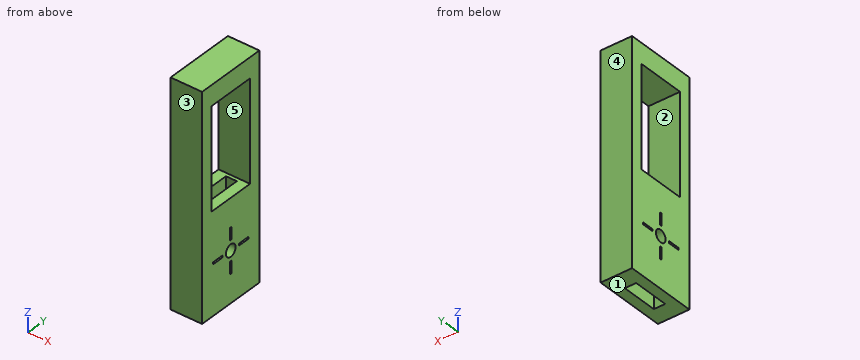
```python
from build123d import *

# Parameters (mm, degrees)
SKETCH1_W           = 17.8
SKETCH1_H           = 25
SKETCH1_R           = 1.5
BOSS_EXTRUDE1_DEPTH = 3.9
SKETCH3_W           = 0.5
SKETCH3_H           = 3
CUT_EXTRUDE1_DEPTH  = 10
CIRPATTERN1_COUNT   = 4
SKETCH4_W           = 2.7
SKETCH4_H           = 10.2
CUT_EXTRUDE2_DEPTH  = 18
SKETCH5_W           = 2.8
SKETCH5_H           = 9
CUT_EXTRUDE3_DEPTH  = 10
SKETCH6_W           = 7.8
SKETCH6_H           = 17.8
BOSS_EXTRUDE2_DEPTH = 30
SKETCH7_W           = 25
SKETCH7_H           = 12
CUT_EXTRUDE4_DEPTH  = 30


with BuildPart() as part:
    # Sketch1 → Boss-Extrude1 (new, symmetric)
    with BuildSketch(Plane.YZ):
        Rectangle(SKETCH1_W, SKETCH1_H)
        with Locations(Location((0, 0, 0), (0, 0, 270))):
            Circle(SKETCH1_R, mode=Mode.SUBTRACT)
    extrude(amount=BOSS_EXTRUDE1_DEPTH, both=True)

    # Sketch3 → Cut-Extrude1 (cut)
    with BuildSketch(Plane(origin=(3.9, 0, 0), x_dir=(0, 0, -1), z_dir=(1, 0, 0))):
        with Locations((0, 4)):
            Rectangle(SKETCH3_W, SKETCH3_H)
    cut_extrude1 = extrude(amount=-CUT_EXTRUDE1_DEPTH, mode=Mode.SUBTRACT)

    # CirPattern1: Cut-Extrude1 ×4 about axis
    cirpattern1_axis = Axis((0, 0, 0), (1, 0, 0))
    for i in range(1, CIRPATTERN1_COUNT):
        add(cut_extrude1.rotate(cirpattern1_axis, i * 360 / CIRPATTERN1_COUNT), mode=Mode.SUBTRACT)

    # Sketch4 → Cut-Extrude2 (cut)
    with BuildSketch(Plane.XY.offset(12.5)):
        Rectangle(SKETCH4_W, SKETCH4_H)
    extrude(amount=-CUT_EXTRUDE2_DEPTH, mode=Mode.SUBTRACT)

    # Sketch5 → Cut-Extrude3 (cut)
    with BuildSketch(Plane(origin=(0, 0, -12.5), x_dir=(-1, 0, 0), z_dir=(0, 0, -1))):
        Rectangle(SKETCH5_W, SKETCH5_H)
    extrude(amount=-CUT_EXTRUDE3_DEPTH, mode=Mode.SUBTRACT)

    # Sketch6 → Boss-Extrude2 (add)
    with BuildSketch(Plane.XY.offset(12.5)):
        Rectangle(SKETCH6_W, SKETCH6_H)
    extrude(amount=BOSS_EXTRUDE2_DEPTH)

    # Sketch7 → Cut-Extrude4 (cut)
    with BuildSketch(Plane(origin=(3.9, 0, 0), x_dir=(0, 0, -1), z_dir=(1, 0, 0))):
        with Locations((-25, 0)):
            Rectangle(SKETCH7_W, SKETCH7_H)
    extrude(amount=-CUT_EXTRUDE4_DEPTH, mode=Mode.SUBTRACT)


solid = part.part
```
Can you work these out from the model? Positions are in its coordinate system, mm. Face numbers are marked on the shaded views. A direction names the side the tool comes from. Coordinates: 2 decimals unless noted, no trailing zeros. Loops run counter-clockwise (first coordinate to the right, second up) from the corner with the lowest first, then second, coordinate; pieces in that order, holes last. Notation, with made-up numbers: M -7,37 L 0,37 A14 cw 0,43 Z; hole C 75,25 d1. An arc over 180 degrees is marked long. Put each result on its own line as item: value. Start each with the question number.
(1) I need wall thicknesses on probe 1 along Z at (x, y) = (-1.5, 3.75); probe 2 along Y at (x, z) = (3.15, 0); probe 3 along Y at (x, z) = (-2.25, 28.5). Which ranges of each line are inside material? Lowest first, please.
(2) Which directions (+Z, -Z, +X, -X, +Y, -Y) give clear straight access to the entire face, cutting with the end or side of a thin tool? Please do the marked faces 4 and 5.
(3) Imagine slicing it at D-D on x = 2.25. List the corners of the cut face in (y, z) for me.
(4) Imagine slicing it at B-B on y = -2. List the corners of the cut face in (x, z) for me, and give its area (4 significant figures).
(5) Will this pin go through, and if not, where does the flat tip stop? pin 1 Ø4 at (x, y) = (0, 2.5) entering from -Z.
(6) Imagine slicing it at A-A on z = -3.5. List the corners of the cut face in (x, y) for me, and give its area (3 significant figures).
(7) We'd pull the mould along Y, two halves only. Please class the marked faces 1, 2 and 3: +Y half, -Y half, draft (parallel to the pull), parting line (faces both ways), or undercut.
(8) Imagine slicing it at C-C on z = 7. List the corners of the cut face in (x, y) for me, and give its area (3 significant figures).
Worked answers:
1. probe 1: z = -12.5 to -0.25, 0.25 to 12.5, 37.5 to 42.5
1. probe 2: y = -8.9 to -5.5, -2.5 to -1.5, 1.5 to 2.5, 5.5 to 8.9
1. probe 3: y = -8.9 to -6, 6 to 8.9
2. face 4: +Z, -Z, +X, -X, +Y
2. face 5: +X, -X
3. outline: M -8.9,-12.5 L 8.9,-12.5 L 8.9,42.5 L -8.9,42.5 Z; hole M -6,12.5 L 6,12.5 L 6,37.5 L -6,37.5 Z; hole M -5.5,-0.25 L -2.5,-0.25 L -2.5,0.25 L -5.5,0.25 Z; hole C 0,0 d3; hole M -0.25,-5.5 L 0.25,-5.5 L 0.25,-2.5 L -0.25,-2.5 Z; hole M -0.25,2.5 L 0.25,2.5 L 0.25,5.5 L -0.25,5.5 Z; hole M 2.5,-0.25 L 5.5,-0.25 L 5.5,0.25 L 2.5,0.25 Z
4. outline: M -3.9,-12.5 L -1.4,-12.5 L -1.4,-2.5 L -1.35,-2.5 L -1.35,12.5 L -3.9,12.5 Z; M -3.9,37.5 L 3.9,37.5 L 3.9,42.5 L -3.9,42.5 Z; M 1.35,-2.5 L 1.4,-2.5 L 1.4,-12.5 L 3.9,-12.5 L 3.9,12.5 L 1.35,12.5 Z
4. area: 165.5 mm2
5. pin 1: stops at z = -12.5
6. outline: M -3.9,-8.9 L 3.9,-8.9 L 3.9,-0.25 L 1.4,-0.25 L 1.4,-4.5 L 1.35,-4.5 L 1.35,-5.1 L -1.35,-5.1 L -1.35,-4.5 L -1.4,-4.5 L -1.4,-0.25 L -3.9,-0.25 Z; M -3.9,0.25 L -1.4,0.25 L -1.4,4.5 L -1.35,4.5 L -1.35,5.1 L 1.35,5.1 L 1.35,4.5 L 1.4,4.5 L 1.4,0.25 L 3.9,0.25 L 3.9,8.9 L -3.9,8.9 Z
6. area: 108 mm2
7. face 1: draft
7. face 2: undercut
7. face 3: -Y half
8. outline: M -3.9,-8.9 L 3.9,-8.9 L 3.9,8.9 L -3.9,8.9 Z; hole M -1.35,-5.1 L 1.35,-5.1 L 1.35,5.1 L -1.35,5.1 Z
8. area: 111 mm2
